from build123d import *

# Parameters (mm, degrees)
F0_R     = 3
F1_DEPTH = 1


with BuildPart() as f1:
    # F0 (on Right) → F1 (new body)
    with BuildSketch(Plane.YZ):
        with BuildLine():
            Line((169.2397592919, 29.7682959138), (-152.7602405548, 29.7682959138))
            ThreePointArc((-152.7602405548, 29.7682959138), (-142.8607456182, 25.6677908504), (-138.7602405548, 15.7682959138))
            ThreePointArc((-138.7602405548, 15.7682959138), (-142.8607456182, 5.8688009772), (-152.7602405548, 1.7682959138))
            Line((-152.7602405548, 1.7682959138), (169.2397594136, 1.7682959138))
            ThreePointArc((169.2397594136, 1.7682959138), (155.2397594452, 15.7682958529), (169.2397592919, 29.7682959138))
        make_face()
        with Locations((8.2397594452, 15.7682959138)):
            Circle(F0_R, mode=Mode.SUBTRACT)
        with BuildLine():
            ThreePointArc((-138.7602405548, 15.7682959138), (-142.8607456182, 25.6677908504), (-152.7602405548, 29.7682959138))
            ThreePointArc((-152.7602405548, 29.7682959138), (-162.6597354914, 25.6677908504), (-166.7602405548, 15.7682959138))
            ThreePointArc((-166.7602405548, 15.7682959138), (-162.6597354914, 5.8688009772), (-152.7602405548, 1.7682959138))
            ThreePointArc((-152.7602405548, 1.7682959138), (-142.8607456182, 5.8688009772), (-138.7602405548, 15.7682959138))
        make_face()
        with Locations((-152.7602405548, 15.7682959138)):
            Circle(F0_R, mode=Mode.SUBTRACT)
        with BuildLine():
            ThreePointArc((183.2397594452, 15.7682959138), (179.1392543276, 25.6677909046), (169.2397592919, 29.7682959138))
            ThreePointArc((169.2397592919, 29.7682959138), (155.2397594452, 15.7682958529), (169.2397594136, 1.7682959138))
            ThreePointArc((169.2397594136, 1.7682959138), (179.1392543706, 5.868800966), (183.2397594452, 15.7682959138))
        make_face()
        with Locations((169.2397594452, 15.7682959138)):
            Circle(F0_R, mode=Mode.SUBTRACT)
    extrude(amount=F1_DEPTH)


solid = f1.part
Verification items for the finished model (mm, model axes). Give positions to 0.01 mm unless a question says otherwise; leave off trailing zeros. Write each loop counter-clockwise with the first axis right and the second up, starting at its lowest first coordinate (ties: lowest second). Pieces come first, ordered by that corner, then holes. Notation, with made-up numbers: M -29,55 L 28,55 A8 ccw 28,65 Z; hole C 62.5,78 d10. An arc over 180 degrees is marked long. Put each result on its own line as item: value. Start each with the question number.
1. Section check B-B (z = 5.5). Record the cut outline in (x, y), and give its area (3 significant figures).
2. Go/stop test with a flat-tipped pin: pin 1 Ø3.5 at (y, z) = (-152.76, 15.77) entering from +X. Record where the tip stops, or that it passes through.
3. Section check A-A (x = 0.5). Record the cut outline in (y, z), and give its area (3 significant figures).
4. Scan lines: line 1 along Z through (x, y) = (0.65, 8.5); line 2 along Y through (x, z) = (0.1, 3); line 3 along Y through (x, z) = (0.25, 11). Record each from-to range of solid material in increasing order. Write a range as [from, to].
5. Section check C-C (z = 25.5). Record the cut outline in (x, y).
Answer list:
1. outline: M 0,-162.28 L 1,-162.28 L 1,178.76 L 0,178.76 Z
1. area: 341 mm2
2. pin 1: through
3. outline: M -152.76,1.77 L 169.24,1.77 A14 ccw 169.24,29.77 L -152.76,29.77 A14 ccw Z; hole C -152.76,15.77 d6; hole C 8.24,15.77 d6; hole C 169.24,15.77 d6
3. area: 9,550 mm2
4. line 1: [1.77, 12.78], [18.76, 29.77]
4. line 2: [-158.5, 174.98]
4. line 3: [-165.92, 182.4]
5. outline: M 0,-162.82 L 1,-162.82 L 1,179.3 L 0,179.3 Z
